from build123d import *

# Parameters (mm, degrees)
SECSKE_W      = 1.2
SECSKE_H      = 5
INTCUT_DEPTH  = 19.423897525
INTCUTS_COUNT = 12
INTCUTS_ANGLE = 330


with BuildPart() as part:
    # SecSke → Body (revolve)
    with BuildSketch(Plane.XY, mode=Mode.PRIVATE) as body_sk:
        with Locations((-0.6, 10.5)):
            Rectangle(SECSKE_W, SECSKE_H)
    revolve(body_sk.sketch.rotate(Axis((-34.925, 0, 0), (1, 0, 0)), 90), axis=Axis((-34.925, 0, 0), (1, 0, 0)))

    # IntCutSke → IntCut (cut, through all)
    with BuildSketch(Plane(origin=(0, 0, 0), x_dir=(0, 0, -1), z_dir=(1, 0, 0))):
        with BuildLine():
            Line((-0.703083639, 10.726983425), (-1.326257139, 7.483384395))
            ThreePointArc((-1.326257139, 7.483384395), (0, 7.6), (1.326257139, 7.483384395))
            Line((1.326257139, 7.483384395), (0.703083639, 10.726983425))
            ThreePointArc((0.703083639, 10.726983425), (0, 10.75), (-0.703083639, 10.726983425))
        make_face()
    intcut = extrude(amount=-INTCUT_DEPTH, mode=Mode.SUBTRACT)

    # IntCuts: IntCut ×12 about axis
    intcuts_axis = Axis((-34.925, 0, 0), (1, 0, 0))
    for i in range(1, INTCUTS_COUNT):
        add(intcut.rotate(intcuts_axis, i * INTCUTS_ANGLE / (INTCUTS_COUNT - 1)), mode=Mode.SUBTRACT)


solid = part.part
The listing builds one solid part. Answer for the finished solid, in the listing's coordinates (mm). Round coordinates to 2 decimals unless told otherwise and drop trailing zeros. Loops run counter-clockwise (first coordinate to the right, second up) from the corner with the lowest first, then second, coordinate; pieces in that order, holes last. Notation, with made-up numbers: M -4,60.5 L 46,60.5 A22 cw 46,67.5 Z; hole C 10,-31 d5. An arc over 180 degrees is marked long. Return JSON: item names as keys, results as strings.
Q1. Find section C-C, the plane y = -8.25. Determine the outline of the cut face in (x, z).
Results list:
{"outline": "M -1.2,-10.05 L 0,-10.05 L 0,-5.73 L -1.2,-5.73 Z; M -1.2,-3.55 L 0,-3.55 L 0,-1.18 L -1.2,-1.18 Z; M -1.2,1.18 L 0,1.18 L 0,3.55 L -1.2,3.55 Z; M -1.2,5.73 L 0,5.73 L 0,10.05 L -1.2,10.05 Z"}
Q2. The mould has two halves that part along Y. Classify faces 1 (the face through (-0.592, -8.569, 3.827)), 2 (the face through (-0.592, 7.91, -10.316)): released by +Y, released by -Y, zero draft, split by the parting line, or undercut.
Results list:
{"face 1": "undercut", "face 2": "split by the parting line"}
Q3. Find section A-A, the plane y = 0. Determine the outline of the cut face in (x, z), plus the area to 3 significant figures.
Results list:
{"outline": "M -1.2,-13 L 0,-13 L 0,-10.75 L -1.2,-10.75 Z; M -1.2,10.75 L 0,10.75 L 0,13 L -1.2,13 Z", "area": "5.40 mm2"}
Q4. Find the intervals of material crossed by line 1 along Y through (x, z) = (-0.4, -9.25); line 2 along Y through (x, z) = (-0.9, 0.25); line 3 along Z through (x, y) = (-0.45, -8.75), in increasing order. Write a range as from..to.
Results list:
{"line 1": "y = -9.13..-5.48, -4.42..-0.99, 0.99..4.42, 5.48..9.13", "line 2": "y = -13..-10.75, 10.75..13", "line 3": "z = -9.61..-5.91, -3.98..-1.08, 1.08..3.98, 5.91..9.61"}
